Model file for the job. Use its own axes, mm. A direction names the side the tool comes from. Round coordinates to 2 decimals unless told otherwise and drop trailing zeros. Order: outer loops, then holes, each group sorted by start corner. A loop starts at its lowest first (then second) coordinate and runs counter-clockwise, first axis right, second up. Notation, with made-up numbers: M 30.5,50.25 L 62.5,50.25 A20 cw 62.5,77.25 Z; hole C 81,-19.5 d10. An arc over 180 degrees is marked long. Return JSON: item names as keys, results as strings. Group by question number.
Item 1: Slice it at A-A on y = -47.5. Write the cut outline in (x, z).
Item 2: Probe line 1 along Y through (x, z) = (-32.5, 35.6); line 2 along Z through (x, y) = (-33.75, -37.75); line 3 along Y through (x, z) = (-33.5, 35.2). List the from-to ranges inside material, lowest first.
Item 3: Slice it at C-C on y = -39.25. Write the cut outline in (x, z).
Item 4: Which spindle directions (+Z, -Z, +X, -X, +Y, -Y) get a long thin tool onto all of the face, cutting with end or side? Do faces 4 (the face through (-32, -46, 37)), 5 (the face through (-32, -45.5, 36.2)). Say none if no direction does.
Item 5: Pull direction Y, two halves, no side cores. Call faces 1 (the face through (-32, -37, 35.5)), 2 (the face through (-30.7, -28.5, 37)), 3 (the face through (-32, -26.5, 35)): pulls with the +Y half, pulls with the -Y half, needs draft (parallel to the pull), parting line crosses it, or undercut.
Item 6: Pin check, flat tips, straight feed: pin 1 Ø1 at (x, y) = (-31.5, -43) entering from +Z; pin 2 Ø2 at (x, y) = (-32.02, -41.75) entering from -Z. Stop position of each tip, or through.
Item 7: Slice it at B-B on z = 35.7. Write the cut outline in (x, y), then the cut area to 3 significant figures.
Item 8: Slice it at D-D on x = -29.75. Write the cut outline in (y, z).
from build123d import *

# Parameters (mm, degrees)
RETAINER_PLATE_START            = 34.5
SKETCH1_W                       = 7
SKETCH1_H                       = 23
RETAINER_PLATE_DEPTH            = 1
RETAINER_MOUNTING_SPACERS_START = 35.5
SKETCH2_R                       = 2
RETAINER_MOUNTING_SPACERS_DEPTH = 1.5
RETAINER_CLEARANCE_HOLES_START  = 34
SKETCH3_R                       = 1.7
SKETCH3_R_2                     = 1.1
RETAINER_CLEARANCE_HOLES_DEPTH  = 4
CLEAR_END_WALL_START            = 33
SKETCH4_W                       = 15
SKETCH4_H                       = 6.3
CLEAR_END_WALL_DEPTH            = 6


with BuildPart() as part:
    # Sketch1 → Retainer_plate (new body)
    with BuildSketch(Plane.XY.offset(RETAINER_PLATE_START)):
        with Locations((-32.018684277, -38)):
            Rectangle(SKETCH1_W, SKETCH1_H)
    extrude(amount=RETAINER_PLATE_DEPTH)

    # Sketch2 → Retainer_mounting_spacers (add)
    with BuildSketch(Plane.XY.offset(RETAINER_MOUNTING_SPACERS_START)):
        with Locations(Location((-32.018684277, -47.5, 0), (0, 0, 270))):
            Circle(SKETCH2_R)
        with Locations(Location((-32.018684277, -28.5, 0), (0, 0, 90))):
            Circle(SKETCH2_R)
    extrude(amount=RETAINER_MOUNTING_SPACERS_DEPTH)

    # Sketch3 → Retainer_clearance_holes (cut)
    with BuildSketch(Plane.XY.offset(RETAINER_CLEARANCE_HOLES_START)):
        with Locations(Location((-32.018684277, -41.745416557, 0), (0, 0, 180))):
            Circle(SKETCH3_R)
        with Locations(Location((-32.018684277, -34.643402341, 0), (0, 0, 180))):
            Circle(SKETCH3_R)
        with Locations(Location((-32.018684277, -47.5, 0), (0, 0, 180))):
            Circle(SKETCH3_R_2)
        with Locations(Location((-32.018684277, -28.5, 0), (0, 0, 180))):
            Circle(SKETCH3_R_2)
    extrude(amount=RETAINER_CLEARANCE_HOLES_DEPTH, mode=Mode.SUBTRACT)

    # Sketch4 → Clear_end_wall (cut)
    with BuildSketch(Plane.XY.offset(CLEAR_END_WALL_START)):
        with Locations((-32.5, -51.85)):
            Rectangle(SKETCH4_W, SKETCH4_H)
    extrude(amount=CLEAR_END_WALL_DEPTH, mode=Mode.SUBTRACT)


solid = part.part
Output values:
{
 "1": {"outline": "M -35.52,34.5 L -33.12,34.5 L -33.12,37 L -34.02,37 L -34.02,35.5 L -35.52,35.5 Z; M -30.92,34.5 L -28.52,34.5 L -28.52,35.5 L -30.02,35.5 L -30.02,37 L -30.92,37 Z"},
 "2": {"line 1": "-48.7 to -48.49, -46.51 to -45.56, -30.44 to -29.49, -27.51 to -26.56", "line 2": "34.5 to 35.5", "line 3": "-48.7 to -42.58, -40.91 to -35.48, -33.81 to -26.5"},
 "3": {"outline": "M -35.52,34.5 L -28.52,34.5 L -28.52,35.5 L -35.52,35.5 Z"},
 "4": {"face 4": "+Z, +X, -X, +Y, -Y", "face 5": "+Z"},
 "5": {"face 1": "undercut", "face 2": "needs draft", "face 3": "pulls with the +Y half"},
 "6": {"pin 1": "z = 35.5", "pin 2": "through"},
 "7": {"outline": "C -32.02,-28.5 d4; M -33.62,-48.7 L -30.42,-48.7 A2 ccw long Z; hole C -32.02,-47.5 d2.2; hole C -32.02,-28.5 d2.2", "area": "15.7 mm²"},
 "8": {"outline": "M -48.7,34.5 L -26.5,34.5 L -26.5,35.5 L -48.7,35.5 Z"}
}
